from build123d import *

# Parameters (mm, degrees)
SKETCH1_R          = 2.3
EXTRUDE1_DEPTH     = 7
FILLET1_R          = 39
FILLET2_R          = 33
FILLET3_R          = 4
FILLET4_R          = 35
SKETCH2_W          = 32.945688526
SKETCH2_H          = 40
CUT_EXTRUDE1_DEPTH = 4
FILLET5_R          = 4


with BuildPart() as part:
    # Sketch1 → Extrude1 (new body)
    with BuildSketch(Plane.XY):
        with BuildLine():
            Line((-10, 0), (-10, 40))
            Line((-10, 40), (-34.835050164, 94.26528975))
            ThreePointArc((-34.835050164, 94.26528975), (-24.125651083, 131.816849255), (10, 150.797122912))
            Line((10, 150.797122912), (38.123036173, 150.797122912))
            Line((38.123036173, 150.797122912), (10, 40))
            Line((10, 40), (10, 0))
            Line((10, 0), (-10, 0))
        make_face()
        with Locations((0, 30)):
            Circle(SKETCH1_R, mode=Mode.SUBTRACT)
        with Locations((4, 8)):
            Circle(SKETCH1_R, mode=Mode.SUBTRACT)
        with Locations((-4, 8)):
            Circle(SKETCH1_R, mode=Mode.SUBTRACT)
        Polygon((24.273596224, 134.519949949), (0, 51.555620572), (-17.877283618, 84.220450394), (-7.457593377, 119.833740044), align=None, mode=Mode.SUBTRACT)
        with BuildLine():
            Line((32.581459881, 142.069152681), (33.097875117, 144.001331581))
            ThreePointArc((33.097875117, 144.001331581), (-9.474149394, 134.549204992), (-26.175231417, 94.26528975))
            Line((-26.175231417, 94.26528975), (-24.182732091, 94.438340134))
            ThreePointArc((-24.182732091, 94.438340134), (-8.246919268, 133.086649081), (32.581459881, 142.069152681))
        make_face(mode=Mode.SUBTRACT)
    extrude(amount=EXTRUDE1_DEPTH)

    # Fillet1
    fillet1_edges = [part.edges().sort_by_distance(p)[0] for p in [
        (-34.835050164, 94.26528975, 3.5),
    ]]
    fillet(fillet1_edges, radius=FILLET1_R)

    # Fillet2
    fillet2_edges = [part.edges().sort_by_distance(p)[0] for p in [
        (-7.457593377, 119.833740044, 3.5),
        (-17.877283618, 84.220450394, 3.5),
    ]]
    fillet(fillet2_edges, radius=FILLET2_R)

    # Fillet3
    fillet3_edges = [part.edges().sort_by_distance(p)[0] for p in [
        (10, 0, 3.5),
        (-10, 0, 3.5),
        (38.123036173, 150.797122912, 3.5),
        (24.273596224, 134.519949949, 3.5),
        (0, 51.555620572, 3.5),
    ]]
    fillet(fillet3_edges, radius=FILLET3_R)

    # Fillet4
    fillet4_edges = [part.edges().sort_by_distance(p)[0] for p in [
        (-10, 40, 3.5),
        (10, 40, 3.5),
    ]]
    fillet(fillet4_edges, radius=FILLET4_R)

    # Sketch2 → Cut-Extrude1 (cut)
    with BuildSketch(Plane.XY.offset(7)):
        with Locations((-0.117072908, 20)):
            Rectangle(SKETCH2_W, SKETCH2_H)
    extrude(amount=-CUT_EXTRUDE1_DEPTH, mode=Mode.SUBTRACT)

    # Fillet5
    fillet5_edges = [part.edges().sort_by_distance(p)[0] for p in [
        (10.274211948, 40, 5),
        (-10.841473657, 40, 5),
    ]]
    fillet(fillet5_edges, radius=FILLET5_R)


solid = part.part
Build history of the part. All positions in model axes, mm. A direction names the side the tool comes from. Round coordinates to 2 decimals unless told otherwise and drop trailing zeros. Write each loop counter-clockwise with the first axis right and the second up, starting at its lowest first coordinate (ties: lowest second). Pieces come first, ordered by that corner, then holes. Notation, with made-up numbers: (67, 48.25) - (94, 48.25) arc R29 cw to (94, 77.25) - close; hole circle Ø2 at (-23.75, 11). An arc over 180 degrees is marked (long way). Use CSV: the item, a comma, the result in double quotes.
(1) Wall check: line 1 (X direction, y = 8, z = 1.95); line 2 (Y direction, x = -4, z = 0.7); line 3 (X direction, y = 30, z = 0.9). Give the ranges that are in metal, low to high.
Response:
line 1,"-10 to -6.3, -1.7 to 1.7, 6.3 to 10"
line 2,"0 to 5.7, 10.3 to 59.16, 118.82 to 136.25, 138.51 to 147.11"
line 3,"-10 to -2.3, 2.3 to 10"
(2) Band-saw the part on B-B (y = 8). Write the cut outline in (x, z).
Response:
outline,"(-10, 0) - (-6.3, 0) - (-6.3, 3) - (-10, 3) - close; (-1.7, 0) - (1.7, 0) - (1.7, 3) - (-1.7, 3) - close; (6.3, 0) - (10, 0) - (10, 3) - (6.3, 3) - close"
(3) Pin check, flat tips, straight feed: P1, Ø3, axis at x = 0, y = 30, coming from the +Z side; P2, Ø1, axis at y = 73, z = 3.5, coming from the -X side; P3, Ø3.5, axis at y = 27, z = 1, coming from the +X side; P4, Ø0.9, axis at y = 18.5, z = 1, coming from the -X side. Stop position of each tip, or through.
Response:
P1,"through"
P2,"x = -25.33"
P3,"x = 10"
P4,"x = -10"
(4) Band-saw the part on A-A (x = -20.5). Write the cut outline in (y, z), plus the area to 3 significant figures.
Response:
outline,"(62.94, 0) - (116.79, 0) - (116.79, 7) - (62.94, 7) - close; (121.13, 0) - (135.92, 0) - (135.92, 7) - (121.13, 7) - close"
area,"480 mm²"
(5) Band-saw the part on D-D (x = 20). Write the cut outline in (y, z), plus the area to 3 significant figures.
Response:
outline,"(79.4, 0) - (119.91, 0) - (119.91, 7) - (79.4, 7) - close; (130.63, 0) - (143.64, 0) - (143.64, 7) - (130.63, 7) - close; (145.6, 0) - (150.8, 0) - (150.8, 7) - (145.6, 7) - close"
area,"411 mm²"
(6) Band-saw the part on C-C (z = 1.5). Write the cut outline in (x, y).
Response:
outline,"(-33.86, 111.62) arc R39 ccw to (-31.32, 86.59) - (-13.17, 46.94) arc R35 cw to (-10, 32.37) - (-10, 4) arc R4 ccw to (-6, 0) - (6, 0) arc R4 ccw to (10, 4) - (10, 35.63) arc R35 cw to (11.08, 44.24) - (36.86, 145.81) arc R4 ccw to (32.98, 150.8) - (10, 150.8) arc R51.02 ccw to start; hole (-26.18, 94.27) - (-24.18, 94.44) arc R45.13 cw to (32.58, 142.07) - (33.1, 144) arc R47.25 ccw to start; hole (-14.04, 97.34) arc R33 ccw to (-11.31, 72.23) - (-4.64, 60.03) arc R4 ccw to (2.71, 60.82) - (21.8, 126.07) arc R4 ccw to (16.28, 130.82) - (6.14, 126.13) arc R33 ccw to (-11.67, 105.45) - close; hole circle Ø4.6 at (-4, 8); hole circle Ø4.6 at (0, 30); hole circle Ø4.6 at (4, 8)"
(7) Mould opens along Y. For faces 5 (the flat face through (-1, 22, 3)), 6 (the cylindrical face through (-18.467, 137.869, 3.451)), 7 (the flat face through (-7.929, 66.043, 3.451)) say: pulls with the +Y half, pulls with the -Y half, needs draft (parallel to the pull), parting line crosses it, or undercut.
Response:
face 5,"needs draft"
face 6,"pulls with the +Y half"
face 7,"undercut"
(8) 3-axis set-ups, long thin cutter, end or side, ignore diameter. For faces 1 (the cylindrical face through (9.45, 40.91, 5.03)), 2 (the flat face through (10, 20, 1)), 3 (the flat face through (-12.87, 101.34, 3.45)), 4 (the flat face through (-1, 40, 5)): which of +Z, -Z, +X, -X, +Y, -Y reach the whole face in a straight line?
Response:
face 1,"+Z, +X, -Y"
face 2,"+Z, -Z, +X, -Y"
face 3,"+Z, -Z"
face 4,"+Z, +X, -X, -Y"
